Build history of the part. All positions in model axes, mm. A direction names the side the tool comes from. Round coordinates to 2 decimals unless told otherwise and drop trailing zeros. Write each loop counter-clockwise with the first axis right and the second up, starting at its lowest first coordinate (ties: lowest second). Pieces come first, ordered by that corner, then holes.
Item 1: Band-saw the part on B-B, the plane y = -8.75. Write the cut outline in (x, z).
Item 2: Mould opens along Z. For faces 1 (the cylindrical face through (7.96, -0.61, 4.48)), 2 (the flat face through (0, 4, -24)), 3 (the flat face through (-1.181, 9.055, -15.291)), 4 (the flat face through (0, 6, -5)) say: +Z half, -Z half, draft (parallel to the pull), parting line (faces both ways), or undercut.
Item 3: Band-saw the part on D-D, the plane x = -6.5. Write the cut outline in (y, z).
Item 4: Band-saw the part on C-C, the plane x = -3.75. Write the cut outline in (y, z), then the cut area to 3 significant figures.
Item 5: Band-saw the part on A-A, the plane x = 0. Write the cut outline in (y, z).
Item 6: Drop flat-ended pins along their axis: pin 1 Ø1 at (x, y) = (7, -6.5) entering from +Z; pin 2 Ø10 at (x, y) = (1, 10.5) entering from -Z; pin 3 Ø1.7 at (x, y) = (0, 13.5) entering from +Z; pin 4 Ø4 at (x, z) = (-8, -17.5) entering from +Y. Give the stop position or say it passes through.
Item 7: 3-axis set-ups, long thin cutter, end or side, ignore diameter. For faces 5 (the cylindrical face through (0.066, 5.843, -19.045)), 6 (the flat face through (-4.588, 7, -2)), 7 (the flat face through (0, 0, 3)), 8 (the flat face through (4.588, 7, -3)): which of +Z, -Z, +X, -X, +Y, -Y reach the whole face in a straight line?
Item 8: Wall check: probe 1 along Z at (x, y) = (-4.5, 5.5); probe 2 along Z at (x, y) = (11.25, 0); probe 3 along Z at (x, y) = (-1, 11). Give the ranges that are in metal, low to high.
```python
from build123d import *
from build123d.topology import SkipClean

# Parameters (mm, degrees)
SKIZZE2_R                       = 12.5
AUFSATZ_LINEAR_AUSTRAGEN1_DEPTH = 3
SKIZZE3_R                       = 1
AUFSATZ_LINEAR_AUSTRAGEN2_DEPTH = 3
SKIZZE4_W                       = 9.175781616
SKIZZE4_H                       = 15
AUFSATZ_LINEAR_AUSTRAGEN3_DEPTH = 5
SCHNITT_LINEAR_AUSTRAGEN1_DEPTH = 10
SKIZZE6_W                       = 10
SKIZZE6_H                       = 25
AUFSATZ_LINEAR_AUSTRAGEN4_DEPTH = 10
VERRUNDUNG1_R                   = 5
SKIZZE7_R                       = 1.5
AUFSATZ_LINEAR_AUSTRAGEN5_DEPTH = 10


with BuildPart() as part:
    # Skizze2 → Aufsatz-Linear austragen1 (new body)
    with BuildSketch(Plane.XY):
        Circle(SKIZZE2_R)
    extrude(amount=AUFSATZ_LINEAR_AUSTRAGEN1_DEPTH)

    # Skizze3 → Aufsatz-Linear austragen2 (add)
    with BuildSketch(Plane.XY.offset(3)):
        with Locations((0, 8.75)):
            Circle(SKIZZE3_R)
        with Locations((6.187184335, 6.187184335)):
            Circle(SKIZZE3_R)
        with Locations((8.75, 0)):
            Circle(SKIZZE3_R)
        with Locations((6.187184335, -6.187184335)):
            Circle(SKIZZE3_R)
        with Locations((0, -8.75)):
            Circle(SKIZZE3_R)
        with Locations((-6.187184335, -6.187184335)):
            Circle(SKIZZE3_R)
        with Locations((-8.75, 0)):
            Circle(SKIZZE3_R)
        with Locations((-6.187184335, 6.187184335)):
            Circle(SKIZZE3_R)
    extrude(amount=AUFSATZ_LINEAR_AUSTRAGEN2_DEPTH)

    # Skizze4 → Aufsatz-Linear austragen3 (add)
    with BuildSketch(Plane(origin=(0, 0, 0), x_dir=(-1, 0, 0), z_dir=(0, 0, -1))):
        with Locations((0, 7.5)):
            Rectangle(SKIZZE4_W, SKIZZE4_H)
    extrude(amount=AUFSATZ_LINEAR_AUSTRAGEN3_DEPTH)

    # Skizze5 → Schnitt-Linear austragen1 (cut)
    with BuildSketch(Plane(origin=(4.587890808, 0, 0), x_dir=(0, 0, -1), z_dir=(1, 0, 0))):
        Polygon((1, 15), (5, 15), (5, 12), align=None)
    extrude(amount=-SCHNITT_LINEAR_AUSTRAGEN1_DEPTH, mode=Mode.SUBTRACT)

    # Skizze6 → Aufsatz-Linear austragen4 (add)
    with BuildSketch(Plane(origin=(0, 10.08, -7.56), x_dir=(1, 0, 0), z_dir=(0, 0.8, -0.6000000000000001))):
        with Locations((0, -5.7)):
            Rectangle(SKIZZE6_W, SKIZZE6_H)
    extrude(amount=AUFSATZ_LINEAR_AUSTRAGEN4_DEPTH)

    # Verrundung1
    # the kernel refuses this fillet: 5 mm, written as the material it takes off along each edge
    with BuildSketch(Plane(origin=(5, 28.5, 17), x_dir=(0, 0.8, -0.6), z_dir=(0, -0.6000000000000001, -0.8))) as verrundung1_piece_1_section:
        with BuildLine():
            CenterArc((VERRUNDUNG1_R, -VERRUNDUNG1_R), VERRUNDUNG1_R, 90, 90)
            Line((0, -VERRUNDUNG1_R), (0, 0))
            Line((0, 0), (VERRUNDUNG1_R, 0))
        make_face()
    verrundung1_piece_1 = extrude(amount=50, mode=Mode.PRIVATE)
    verrundung1_piece_1 = split(verrundung1_piece_1, bisect_by=Plane(origin=(4.587890808, 18.932165371, 1.027012133), z_dir=(1, 0, 0)), keep=Keep.TOP, mode=Mode.PRIVATE)
    add(verrundung1_piece_1, mode=Mode.SUBTRACT)
    with BuildSketch(Plane(origin=(5, 28.5, 17), x_dir=(0, 0.8, -0.6), z_dir=(0, -0.6000000000000001, -0.8))) as verrundung1_piece_2_section:
        with BuildLine():
            CenterArc((VERRUNDUNG1_R, -VERRUNDUNG1_R), VERRUNDUNG1_R, 90, 90)
            Line((0, -VERRUNDUNG1_R), (0, 0))
            Line((0, 0), (VERRUNDUNG1_R, 0))
        make_face()
    verrundung1_piece_2 = extrude(amount=50, mode=Mode.PRIVATE)
    verrundung1_piece_2 = split(verrundung1_piece_2, bisect_by=Plane(origin=(3.559847319, 15, 2.011430888), z_dir=(0, 1, 0)), keep=Keep.TOP, mode=Mode.PRIVATE)
    add(verrundung1_piece_2, mode=Mode.SUBTRACT)
    with BuildSketch(Plane(origin=(5, 28.5, 17), x_dir=(0, 0.8, -0.6), z_dir=(0, -0.6000000000000001, -0.8))) as verrundung1_piece_3_section:
        with BuildLine():
            CenterArc((VERRUNDUNG1_R, -VERRUNDUNG1_R), VERRUNDUNG1_R, 90, 90)
            Line((0, -VERRUNDUNG1_R), (0, 0))
            Line((0, 0), (VERRUNDUNG1_R, 0))
        make_face()
    verrundung1_piece_3 = extrude(amount=50, mode=Mode.PRIVATE)
    verrundung1_piece_3 = split(verrundung1_piece_3, bisect_by=Plane(origin=(3.543313448, 9.872718636, -5), z_dir=(0, 0, -1)), keep=Keep.TOP, mode=Mode.PRIVATE)
    add(verrundung1_piece_3, mode=Mode.SUBTRACT)
    with BuildSketch(Plane(origin=(-5, -1.5, -23), x_dir=(0, 0.7999999999999999, -0.6000000000000001), z_dir=(0, 0.6000000000000001, 0.8))) as verrundung1_piece_4_section:
        with BuildLine():
            CenterArc((VERRUNDUNG1_R, -VERRUNDUNG1_R), VERRUNDUNG1_R, 90, 90)
            Line((0, -VERRUNDUNG1_R), (0, 0))
            Line((0, 0), (VERRUNDUNG1_R, 0))
        make_face()
    verrundung1_piece_4 = extrude(amount=50, mode=Mode.PRIVATE)
    verrundung1_piece_4 = split(verrundung1_piece_4, bisect_by=Plane(origin=(-4.807563365, 10.769431466, -5), z_dir=(0, 0, -1)), keep=Keep.TOP, mode=Mode.PRIVATE)
    add(verrundung1_piece_4, mode=Mode.SUBTRACT)
    with BuildSketch(Plane(origin=(-5, -1.5, -23), x_dir=(0, 0.7999999999999999, -0.6000000000000001), z_dir=(0, 0.6000000000000001, 0.8))) as verrundung1_piece_5_section:
        with BuildLine():
            CenterArc((VERRUNDUNG1_R, -VERRUNDUNG1_R), VERRUNDUNG1_R, 90, 90)
            Line((0, -VERRUNDUNG1_R), (0, 0))
            Line((0, 0), (VERRUNDUNG1_R, 0))
        make_face()
    verrundung1_piece_5 = extrude(amount=50, mode=Mode.PRIVATE)
    verrundung1_piece_5 = split(verrundung1_piece_5, bisect_by=Plane(origin=(-4.587890808, 14, -3.666666667), z_dir=(-1, 0, 0)), keep=Keep.TOP, mode=Mode.PRIVATE)
    add(verrundung1_piece_5, mode=Mode.SUBTRACT)
    with BuildSketch(Plane(origin=(-5, -1.5, -23), x_dir=(0, 0.7999999999999999, -0.6000000000000001), z_dir=(0, 0.6000000000000001, 0.8))) as verrundung1_piece_6_section:
        with BuildLine():
            CenterArc((VERRUNDUNG1_R, -VERRUNDUNG1_R), VERRUNDUNG1_R, 90, 90)
            Line((0, -VERRUNDUNG1_R), (0, 0))
            Line((0, 0), (VERRUNDUNG1_R, 0))
        make_face()
    verrundung1_piece_6 = extrude(amount=50, mode=Mode.PRIVATE)
    verrundung1_piece_6 = split(verrundung1_piece_6, bisect_by=Plane(origin=(-3.559847319, 15, 2.011430888), z_dir=(0, 1, 0)), keep=Keep.TOP, mode=Mode.PRIVATE)
    add(verrundung1_piece_6, mode=Mode.SUBTRACT)
    with BuildSketch(Plane(origin=(-5, 6.5, -29), x_dir=(0, -0.8, 0.6), z_dir=(0, 0.6000000000000001, 0.8)), Plane(origin=(5, 36.5, 11), x_dir=(0, -0.8, 0.6), z_dir=(0, -0.6000000000000001, -0.8))) as verrundung1_piece_7:
        with BuildLine():
            CenterArc((VERRUNDUNG1_R, VERRUNDUNG1_R), VERRUNDUNG1_R, 180, 90)
            Line((0, VERRUNDUNG1_R), (0, 0))
            Line((0, 0), (VERRUNDUNG1_R, 0))
        make_face()
    extrude(amount=50, mode=Mode.SUBTRACT)

    # Skizze7 → Aufsatz-Linear austragen5 (add)
    with SkipClean():  # the faces are left unmerged after this step: merging them gives an invalid solid
        with BuildSketch(Plane(origin=(0, -4.08, -5.44), x_dir=(-1, 0, 0), z_dir=(0, -0.6000000000000002, -0.7999999999999999))):
            with Locations(Location((0, 17.6, 0), (0, 0, 90))):
                Circle(SKIZZE7_R)
        extrude(amount=AUFSATZ_LINEAR_AUSTRAGEN5_DEPTH)


solid = part.part
```
Results:
1. outline: (-8.93, 0) - (8.93, 0) - (8.93, 3) - (1, 3) - (1, 6) - (-1, 6) - (-1, 3) - (-8.93, 3) - close
2. face 1: draft
2. face 2: -Z half
2. face 3: undercut
2. face 4: undercut
3. outline: (-10.68, 0) - (10.68, 0) - (10.68, 3) - (7.14, 3) - (7.14, 6) - (5.24, 6) - (5.24, 3) - (-5.24, 3) - (-5.24, 6) - (-7.14, 6) - (-7.14, 3) - (-10.68, 3) - close
4. outline: (-11.92, 0) - (0, 0) - (0, -5) - (14.12, -5) - (7.35, -14.02) - (12.65, -17.98) - (27.65, 2.02) - (22.35, 5.98) - (15, -3.82) - (15, 0) - (11.92, 0) - (11.92, 3) - (-11.92, 3) - close
4. area: 311 mm2
5. outline: (-12.5, 0) - (0, 0) - (0, -5) - (12, -5) - (6, -13) - (8.8, -15.1) - (2.8, -23.1) - (5.2, -24.9) - (11.2, -16.9) - (14, -19) - (29, 1) - (21, 7) - (15, -1) - (15, 0) - (12.5, 0) - (12.5, 3) - (9.75, 3) - (9.75, 6) - (7.75, 6) - (7.75, 3) - (-7.75, 3) - (-7.75, 6) - (-9.75, 6) - (-9.75, 3) - (-12.5, 3) - close
6. pin 1: stops at z = 6
6. pin 2: stops at z = -24.39
6. pin 3: stops at z = 0
6. pin 4: passes through
7. face 5: none
7. face 6: -X, -Y
7. face 7: +Z
7. face 8: +X, -Y
8. probe 1: z = -5 to 3
8. probe 2: z = 0 to 3
8. probe 3: z = -16.75 to -6.5, -5 to 3
